Geometry check sheet. Reference: the model listing, model coordinates, mm. Face numbers are marked on the shaded views. Give positions to 0.01 mm unless a question says otherwise; leave off trailing zeros. Loops run counter-clockwise (first coordinate to the right, second up) from the corner with the lowest first, then second, coordinate; pieces in that order, holes last. Notation, with made-up numbers: (-9.5, 7) - (30.5, 7) arc R15 cw to (30.5, 25) - close; hole circle Ø7 at (5.25, 64.25). An arc over 180 degrees is marked (long way). Use a Markdown table: item, result. Add a question column.
1. Material ranges on L1, parallel to X at y = -11, z = 1; L2, parallel to X at y = 2, z = 3.55; L3, parallel to X at y = -24.5, z = 2.1, recorded low to high.
2. Draft check along X on the marked faces 1, 2, 3 and 4. Enter one of: pulls with the +X half, pulls with the -X half, needs draft (parallel to the pull), parting line crosses it, or undercut.
3. Cross-section at D-D on z = 0.8. Count the separate pieces of the cut face and the enclosed holes in it, and give its area (3 significant figures).
4. Cross-section at B-B on x = -33. Enter the section's corners in (y, z).
5. Cross-section at A-A on y = 23.5. Enter the section's corners in (x, z), and give its area (4 significant figures).
6. Cross-section at C-C on y = 6. Enter the section's corners in (x, z), and give its area (3 significant figures).
7. Depth check by flat-ended pin: P1, Ø3, axis at y = 32.5, z = 3, coming from the -X side; P2, Ø2.5, axis at x = 0, y = -12, coming from the +Z side; P3, Ø1.5, axis at y = 29.5, z = 3, coming from the -X side; P4, Ø2, axis at y = -1, z = 3.5, coming from the +X side. Enter the tip coordinate at first touch or a pass-through.
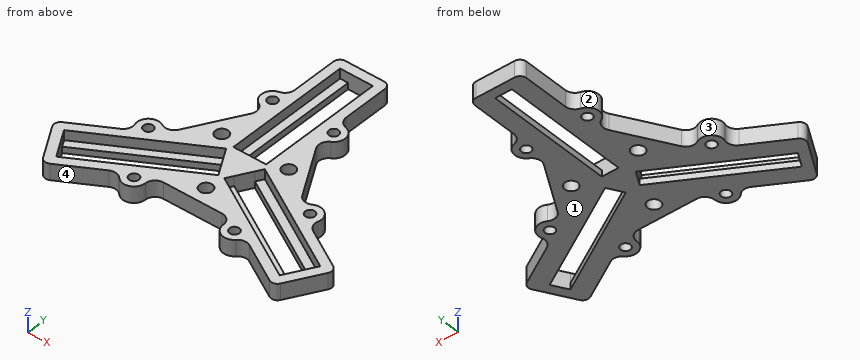
from build123d import *

# Parameters (mm, degrees)
SKETCH1_W           = 5.2
SKETCH1_H           = 39
BOSS_EXTRUDE1_DEPTH = 5
SKETCH2_W           = 10.2
SKETCH2_H           = 39
CUT_EXTRUDE1_DEPTH  = 3.05
CUT_EXTRUDE2_REACH  = 65.739
SKETCH3_R           = 2
SKETCH4_R           = 3.5
SKETCH4_R_2         = 1.5
BOSS_EXTRUDE2_DEPTH = 5
FILLET1_R           = 3
FILLET2_R           = 3
FILLET3_R           = 2


with BuildPart() as part:
    # Sketch1 → Boss-Extrude1 (new body)
    with BuildSketch(Plane.XY):
        Polygon((-8, 46), (8, 46), (8, 20), (21.320508076, -3.07179677), (43.837168574, -16.07179677), (35.837168574, -29.92820323), (13.320508076, -16.92820323), (-13.320508076, -16.92820323), (-35.837168574, -29.92820323), (-43.837168574, -16.07179677), (-21.320508076, -3.07179677), (-8, 20), align=None)
        Polygon((4.764101615, 0.25166605), (2.164101615, -4.25166605), (35.939092363, -23.75166605), (38.539092363, -19.24833395), align=None, mode=Mode.SUBTRACT)
        with Locations((0, 23.5)):
            Rectangle(SKETCH1_W, SKETCH1_H, mode=Mode.SUBTRACT)
        Polygon((-2.164101615, -4.25166605), (-4.764101615, 0.25166605), (-38.539092363, -19.24833395), (-35.939092363, -23.75166605), align=None, mode=Mode.SUBTRACT)
    extrude(amount=BOSS_EXTRUDE1_DEPTH)

    # Sketch2 → Cut-Extrude1 (cut)
    with BuildSketch(Plane.XY.offset(5)):
        with Locations((0, 23.5)):
            Rectangle(SKETCH2_W, SKETCH2_H)
        Polygon((39.789092363, -17.083270441), (34.689092363, -25.916729559), (0.914101615, -6.416729559), (6.014101615, 2.416729559), align=None)
        Polygon((-34.689092363, -25.916729559), (-39.789092363, -17.083270441), (-6.014101615, 2.416729559), (-0.914101615, -6.416729559), align=None)
    extrude(amount=-CUT_EXTRUDE1_DEPTH, mode=Mode.SUBTRACT)

    # Sketch3 → Cut-Extrude2 (cut, up to next)
    with BuildSketch(Plane.XY.offset(5), mode=Mode.PRIVATE) as cut_extrude2_sk1:
        with Locations((0, -12)):
            Circle(SKETCH3_R)
    cut_extrude2_tool1 = extrude(cut_extrude2_sk1.sketch, amount=-CUT_EXTRUDE2_REACH, mode=Mode.PRIVATE) & part.part
    # Sketch3 → Cut-Extrude2 (cut, up to next)
    with BuildSketch(Plane.XY.offset(5), mode=Mode.PRIVATE) as cut_extrude2_sk2:
        with Locations((-10.392304845, 6)):
            Circle(SKETCH3_R)
    cut_extrude2_tool2 = extrude(cut_extrude2_sk2.sketch, amount=-CUT_EXTRUDE2_REACH, mode=Mode.PRIVATE) & part.part
    # Sketch3 → Cut-Extrude2 (cut, up to next)
    with BuildSketch(Plane.XY.offset(5), mode=Mode.PRIVATE) as cut_extrude2_sk3:
        with Locations((10.392304845, 6)):
            Circle(SKETCH3_R)
    cut_extrude2_tool3 = extrude(cut_extrude2_sk3.sketch, amount=-CUT_EXTRUDE2_REACH, mode=Mode.PRIVATE) & part.part
    add(cut_extrude2_tool1.solids().sort_by_distance((0, -12, 5))[0], mode=Mode.SUBTRACT)
    add(cut_extrude2_tool2.solids().sort_by_distance((-10.392305, 6, 5))[0], mode=Mode.SUBTRACT)
    add(cut_extrude2_tool3.solids().sort_by_distance((10.392305, 6, 5))[0], mode=Mode.SUBTRACT)

    # Sketch4 → Boss-Extrude2 (add)
    # profile 1 of 6: a face of its own
    with BuildSketch(Plane.XY.offset(5)):
        with Locations((9.5, 23.5)):
            Circle(SKETCH4_R)
        with Locations((9.5, 23.5)):
            Circle(SKETCH4_R_2, mode=Mode.SUBTRACT)
    # profile 2 of 6: a face of its own
    with BuildSketch(Plane.XY.offset(5)):
        with Locations((-9.5, 23.5)):
            Circle(SKETCH4_R)
        with Locations((-9.5, 23.5)):
            Circle(SKETCH4_R_2, mode=Mode.SUBTRACT)
    # profile 3 of 6: a face of its own
    with BuildSketch(Plane.XY.offset(5)):
        with Locations((25.101596989, -3.522758664)):
            Circle(SKETCH4_R)
        with Locations((25.101596989, -3.522758664)):
            Circle(SKETCH4_R_2, mode=Mode.SUBTRACT)
    # profile 4 of 6: a face of its own
    with BuildSketch(Plane.XY.offset(5)):
        with Locations((15.601596989, -19.977241336)):
            Circle(SKETCH4_R)
        with Locations((15.601596989, -19.977241336)):
            Circle(SKETCH4_R_2, mode=Mode.SUBTRACT)
    # profile 5 of 6: a face of its own
    with BuildSketch(Plane.XY.offset(5)):
        with Locations((-15.601596989, -19.977241336)):
            Circle(SKETCH4_R)
        with Locations((-15.601596989, -19.977241336)):
            Circle(SKETCH4_R_2, mode=Mode.SUBTRACT)
    # profile 6 of 6: a face of its own
    with BuildSketch(Plane.XY.offset(5)):
        with Locations((-25.101596989, -3.522758664)):
            Circle(SKETCH4_R)
        with Locations((-25.101596989, -3.522758664)):
            Circle(SKETCH4_R_2, mode=Mode.SUBTRACT)
    extrude(amount=-BOSS_EXTRUDE2_DEPTH)

    # Fillet1
    # the kernel refuses this fillet: 3 mm, written as the material it adds along each edge
    with BuildSketch(Plane(origin=(8, 26.66227766, 0), x_dir=(0.9944903161976937, 0.10482848367219241, 0), z_dir=(0, 0, 1)), Plane(origin=(19.090209776, -20.25934206, 0), x_dir=(-0.40646102819849994, -0.9136681194809295, 0), z_dir=(0, 0, 1)), Plane(origin=(-27.090209776, -6.4029356, 0), x_dir=(-0.5880292879992107, 0.8088396358086942, 0), z_dir=(0, 0, 1))) as fillet1_piece_1:
        with BuildLine():
            CenterArc((3.314967721, 2.830369059), FILLET1_R, 173.982715136, 76.657636203)
            Line((0.331496772, 3.14485451), (0.271827353, 3.151144219))
            Line((0.271827353, 3.151144219), (-0.059669419, 0.006289709))
            Line((-0.059669419, 0.006289709), (0.019889806, -0.056607381))
            ThreePointArc((0.019889806, -0.056607381), (1.160238702, 0.137902764), (2.300587598, -0.056607381))
            Line((2.300587598, -0.056607381), (2.320477404, 0))
        make_face()
    extrude(amount=5)
    with BuildSketch(Plane(origin=(8, 20.33772234, 0), x_dir=(0, -1, 0), z_dir=(0, 0, 1)), Plane(origin=(13.612984201, -17.0970644, 0), x_dir=(-0.8660254037844379, 0.5000000000000013, 0), z_dir=(0, 0, 1)), Plane(origin=(-21.612984201, -3.24065794, 0), x_dir=(0.8660254037844385, 0.5000000000000004, 0), z_dir=(0, 0, 1))) as fillet1_piece_2:
        with BuildLine():
            CenterArc((3.27592086, 0.605796547), FILLET1_R, 172.092756849, 19.557213735)
            Line((0.30444462, 1.018505833), (0.245015095, 1.026760019))
            ThreePointArc((0.245015095, 1.026760019), (0.133629185, 0.514810643), (-0.054210474, 0.025714286))
            Line((-0.054210474, 0.025714286), (0, -0.06))
            ThreePointArc((0, -0.06), (0.16886117, -0.06), (0.278958369, -0.012115931))
            Line((0.278958369, -0.012115931), (0.33772234, 0))
        make_face()
    extrude(amount=5)
    with BuildSketch(Plane(origin=(-8, 20.33772234, 0), x_dir=(-0.9581124549425506, -0.2863922549301202, 0), z_dir=(0, 0, 1)), Plane(origin=(21.612984201, -3.24065794, 0), x_dir=(0.231033259254711, 0.9729458531275754, 0), z_dir=(0, 0, 1)), Plane(origin=(-13.612984201, -17.0970644, 0), x_dir=(0.7270791956878222, -0.6865535981975109, 0), z_dir=(0, 0, 1))) as fillet1_piece_3:
        with BuildLine():
            CenterArc((1.518619579, 2.965205138), FILLET1_R, 241.707941077, 19.557213735)
            Line((0.096721062, 0.32357598), (0.068283092, 0.270743397))
            ThreePointArc((0.068283092, 0.270743397), (-0.009126216, 0.178971525), (-0.057486747, 0.017183535))
            Line((-0.057486747, 0.017183535), (0.009111717, -0.059304103))
            ThreePointArc((0.009111717, -0.059304103), (0.531516853, -0.019405995), (1.053921988, -0.059304103))
            Line((1.053921988, -0.059304103), (1.063033705, 0))
        make_face()
    extrude(amount=5)
    with BuildSketch(Plane(origin=(-8, 26.66227766, 0), x_dir=(-0.9944903161976939, 0.10482848367219239, 0), z_dir=(0, 0, 1))) as fillet1_piece_4:
        with BuildLine():
            CenterArc((3.314967721, -2.830369059), FILLET1_R, 109.359648661, 76.657636203)
            Line((0.331496772, -3.14485451), (0.271827353, -3.151144219))
            Line((0.271827353, -3.151144219), (-0.059669419, -0.006289709))
            Line((-0.059669419, -0.006289709), (0.019889806, 0.056607381))
            ThreePointArc((0.019889806, 0.056607381), (1.160238702, -0.137902764), (2.300587598, 0.056607381))
            Line((2.300587598, 0.056607381), (2.320477404, 0))
        make_face()
    extrude(amount=5)
    with BuildSketch(Plane(origin=(27.090209776, -6.4029356, 0), x_dir=(0.8660254037844388, -0.4999999999999998, 0), z_dir=(0, 0, 1)), Plane(origin=(-19.090209776, -20.25934206, 0), x_dir=(-0.8660254037844379, -0.5000000000000012, 0), z_dir=(0, 0, 1))) as fillet1_piece_5:
        with BuildLine():
            CenterArc((3.16227766, 3), FILLET1_R, 193.342363797, 76.657636203)
            Line((0.243252128, 2.307692308), (0.184871617, 2.293846154))
            ThreePointArc((0.184871617, 2.293846154), (0.258769028, 1.139390016), (-0.054210474, 0.025714286))
            Line((-0.054210474, 0.025714286), (0, -0.06))
            Line((0, -0.06), (3.16227766, -0.06))
            Line((3.16227766, -0.06), (3.16227766, 0))
        make_face()
    extrude(amount=5)

    # Fillet2
    fillet2_edges = [part.edges().sort_by_distance(p)[0] for p in [
        (8, 20, 2.5),
    ]]
    fillet(fillet2_edges, radius=FILLET2_R)
    fillet2_2_edges = [part.edges().sort_by_distance(p)[0] for p in [
        (-13.320508076, -16.92820323, 2.5),
    ]]
    fillet(fillet2_2_edges, radius=FILLET2_R)
    fillet2_3_edges = [part.edges().sort_by_distance(p)[0] for p in [
        (13.320508076, -16.92820323, 2.5),
    ]]
    fillet(fillet2_3_edges, radius=FILLET2_R)
    fillet2_4_edges = [part.edges().sort_by_distance(p)[0] for p in [
        (-8, 20, 2.5),
    ]]
    fillet(fillet2_4_edges, radius=FILLET2_R)
    fillet2_5_edges = [part.edges().sort_by_distance(p)[0] for p in [
        (-21.320508076, -3.07179677, 2.5),
    ]]
    fillet(fillet2_5_edges, radius=FILLET2_R)
    fillet2_6_edges = [part.edges().sort_by_distance(p)[0] for p in [
        (21.320508076, -3.07179677, 2.5),
    ]]
    fillet(fillet2_6_edges, radius=FILLET2_R)

    # Fillet3
    fillet3_edges = [part.edges().sort_by_distance(p)[0] for p in [
        (43.837168574, -16.07179677, 2.5),
        (35.837168574, -29.92820323, 2.5),
        (-35.837168574, -29.92820323, 2.5),
        (-43.837168574, -16.07179677, 2.5),
        (-8, 46, 2.5),
        (8, 46, 2.5),
    ]]
    fillet(fillet3_edges, radius=FILLET3_R)


solid = part.part
Values found:
| question | item | result |
|---|---|---|
| 1 | L1 | x = -35.05 to -24.25, -13.85 to -1.73, 1.73 to 13.85, 24.25 to 35.05 |
| 1 | L2 | x = -18.39 to -6.74, -5.77 to 5.77, 6.74 to 18.39 |
| 1 | L3 | x = -38.97 to -35.51, -32.24 to -26.44, 26.44 to 32.24, 35.51 to 38.97 |
| 2 | face 1 | needs draft |
| 2 | face 2 | pulls with the -X half |
| 2 | face 3 | undercut |
| 2 | face 4 | undercut |
| 3 | separate pieces | 1 |
| 3 | enclosed holes | 12 |
| 3 | area | 1,920 mm2 |
| 4 | outline | (-28.29, 0) - (-22.05, 0) - (-22.05, 1.95) - (-24.94, 1.95) - (-24.94, 5) - (-28.29, 5) - close; (-16.05, 0) - (-9.81, 0) - (-9.81, 5) - (-13.16, 5) - (-13.16, 1.95) - (-16.05, 1.95) - close |
| 5 | outline | (-13, 0) - (-11, 0) - (-11, 5) - (-13, 5) - close; (-8, 0) - (-2.6, 0) - (-2.6, 1.95) - (-5.1, 1.95) - (-5.1, 5) - (-8, 5) - close; (2.6, 0) - (8, 0) - (8, 5) - (5.1, 5) - (5.1, 1.95) - (2.6, 1.95) - close; (11, 0) - (13, 0) - (13, 5) - (11, 5) - close |
| 5 | area | 58.75 mm2 |
| 6 | outline | (-16.08, 0) - (-12.39, 0) - (-12.39, 5) - (-16.08, 5) - close; (-8.39, 0) - (-2.6, 0) - (-2.6, 1.95) - (-5.1, 1.95) - (-5.1, 5) - (-8.39, 5) - close; (2.6, 0) - (8.39, 0) - (8.39, 5) - (5.1, 5) - (5.1, 1.95) - (2.6, 1.95) - close; (12.39, 0) - (16.08, 0) - (16.08, 5) - (12.39, 5) - close |
| 6 | area | 79.6 mm2 |
| 7 | P1 | stops at x = -8 |
| 7 | P2 | passes through |
| 7 | P3 | stops at x = -8.2 |
| 7 | P4 | stops at x = 28.25 |
